Autodesk Inventor part; units mm, degrees
ref_plane "YZ Plane" through (0, 0, 0) normal (1, 0, 0) x (0, 1, 0)
ref_plane "XZ Plane" through (0, 0, 0) normal (0, 1, 0) x (-1, 0, 0)
ref_plane "XY Plane" through (0, 0, 0) normal (0, 0, 1) x (1, 0, 0)
sketch "Skizze1" plane through (0, 0, 0) normal (0, 0, 1) x (1, 0, 0)
  line L0 (-6, 8.3) -> (6, 8.3)
  line L1 (0, 0) -> (0, 8.3) construction
  line L2 (-6, 8.3) -> (-6, 4.0788)
  circle A0 centre (0, -15) radius 20 construction
  line L3 (6, 8.3) -> (6, 4.0788)
  line L4 (-6, 4.0788) -> (6, 4.0788) construction
  line L5 (-13.2288, 0) -> (13.2288, 0)
  arc A1 (-6, 4.0788) -> (-13.2288, 0) centre (0, -15) ccw
  arc A2 (13.2288, 0) -> (6, 4.0788) centre (0, -15) ccw
  point P0 (0, 5)
  dimension "d0" = 40
  dimension "d1" = 12
  dimension "d2" = 3.3
  dimension "d3" = 5
extrude "Extrusion1" add sketch "Skizze1" along normal blind 15
equation "\"d0\" = D"
equation "\"d1\" = Passfeder_Width_40"
equation "\"D\" = 40"
properties part number "Capston_Disc_Flachstelle"
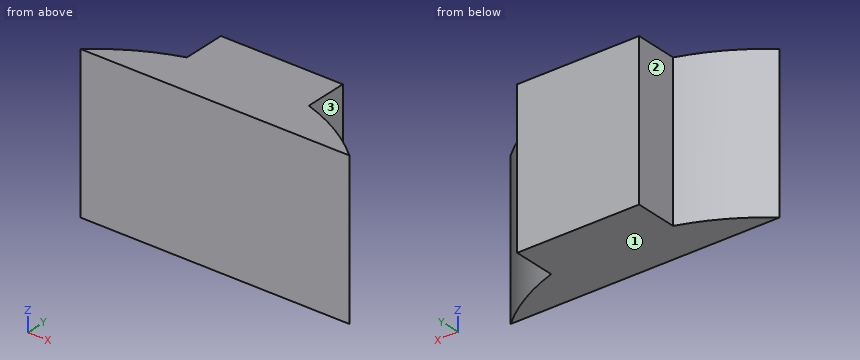
Check sheet for the modelled part. Datum: model origin and axes. Units: mm. Face numbers are marked on the shaded views. A direction names the side the tool comes from. Round coordinates to 2 decimals unless told otherwise and drop trailing zeros. Order: outer loops, then holes, each group sorted by start corner. A loop starts at its lowest first (then second) coordinate and runs counter-clockwise, first axis right, second up.
1) Section check B-B (y = 5). Record the boundary of the cut face in (x, z), and give its area (3 significant figures).
2) Go/stop test with flat-tipped pins: pin 1 Ø1.3 at (y, z) = (7, 7) entering from -X; pin 2 Ø4.5 at (y, z) = (7, 7.5) entering from +X; pin 3 Ø1.5 at (y, z) = (2, 6) entering from +X. Record where each tip stops, or that it passes through.
3) Section check A-A (z = 14.25). Record the boundary of the cut face in (x, y), and give its area (3 significant figures).
4) Tool access check on the marked faces 1, 2 and 3. Record the directions out of +Z, -Z, +X, -X, +Y, -Y that give a thin tool (end or side, any length) a straight path to the whole face; none if there is none.
5) Section check C-C (x = -11.5). Record the boundary of the cut face in (y, z), and give its area (3 significant figures).
6) Scan lines: line 1 (X direction, y = 7, z = 3.5); line 2 (Y direction, x = 9.5, z = 3.75); line 3 (X direction, y = 2.25, z = 7). Record each from-to range of solid material in increasing order.
Result:
1. outline: (-6, 0) - (6, 0) - (6, 15) - (-6, 15) - close
1. area: 180 mm2
2. pin 1: stops at x = -6
2. pin 2: stops at x = 6
2. pin 3: stops at x = 11.66
3. outline: (-13.23, 0) - (13.23, 0) arc R20 ccw to (6, 4.08) - (6, 8.3) - (-6, 8.3) - (-6, 4.08) arc R20 ccw to start
3. area: 134 mm2
4. face 1: -Z, +X, -X, +Y, -Y
4. face 2: +Z, -Z, -X, +Y
4. face 3: +Z, -Z, +X, +Y
5. outline: (0, 0) - (1.36, 0) - (1.36, 15) - (0, 15) - close
5. area: 20.4 mm2
6. line 1: x = -6 to 6
6. line 2: y = 0 to 2.6
6. line 3: x = -10.12 to 10.12
